from build123d import *

# Parameters (mm, degrees)
ESTRUSIONE_ESTRUSIONE1_DEPTH           = 20
SCHIZZO2_R                             = 3.15
TAGLIO_ESTRUSIONE1_DEPTH               = 0.5
FORO_SVASATO_PER_VITE_M3_1_D           = 3.4
FORO_SVASATO_PER_VITE_M3_1_CSINK_D     = 6.3
FORO_SVASATO_PER_VITE_M3_1_CSINK_ANGLE = 90


with BuildPart() as part:
    # Schizzo1 → Estrusione-Estrusione1 (new body)
    with BuildSketch(Plane.XY):
        with BuildLine():
            Line((7.2, -12.4), (-7.2, -12.4))
            Line((-7.2, -12.4), (-7.2, -15.4))
            ThreePointArc((-7.2, -15.4), (0, -16.607910427), (7.2, -15.4))
            Line((7.2, -15.4), (7.2, -12.4))
        make_face()
    extrude(amount=-ESTRUSIONE_ESTRUSIONE1_DEPTH)

    # Schizzo2 → Taglio-Estrusione1 (cut)
    with BuildSketch(Plane(origin=(0, -16.607910427, 0), x_dir=(-1, 0, 0), z_dir=(0, -1, 0))):
        with Locations((0, 13.333333333)):
            Circle(SCHIZZO2_R)
        with Locations((0, 6.666666667)):
            Circle(SCHIZZO2_R)
    extrude(amount=-TAGLIO_ESTRUSIONE1_DEPTH, mode=Mode.SUBTRACT)

    # Foro svasato per Vite M3-1 (through all)
    with Locations(Plane(origin=(0, -16.107910427, -6.666666667), x_dir=(-1, 0, 0), z_dir=(0, -1, 0))):
        with Locations((0, 0), (0, 6.666666666)):
            CounterSinkHole(FORO_SVASATO_PER_VITE_M3_1_D / 2, FORO_SVASATO_PER_VITE_M3_1_CSINK_D / 2, counter_sink_angle=FORO_SVASATO_PER_VITE_M3_1_CSINK_ANGLE)


solid = part.part
Part model, mm, in its own coordinate system. A direction names the side the tool comes from. Coordinates: 2 decimals unless noted, no trailing zeros. Loops run counter-clockwise (first coordinate to the right, second up) from the corner with the lowest first, then second, coordinate; pieces in that order, holes last. Notation, with made-up numbers: (-18, 86) - (22, 86) arc R11 ccw to (22, 100) - close; hole circle Ø2 at (-8.5, 37.25). An arc over 180 degrees is marked (long way). Write each question's results on one line, items separated by ' | '. Start each with the question number.
Q1. Slice it at B-B on y = -12.8. Give the cut face in (x, z), and give its area (3 significant figures).
Q2. Two-plate mould, pull along X, no slides. Class faces 1 (the cylindrical face through (-1.73, -16.54, -9.86)), 2 (the cylindrical face through (-0.369, -13.513, -11.674)), 3 (the flat face through (0, -12.4, -10)): +X half, -X half, draft (parallel to the pull), parting line (faces both ways), or undercut.
Q3. Slice it at A-A on x = 0. Give the cut face in (y, z), and give its area (3 significant figures).
Q4. Slice it at C-C on x = 4. Give the cut face in (y, z), and give its area (3 significant figures).
Q5. Drop flat-ended pins along their axis: pin 1 Ø4 at (x, z) = (0, -6.67) entering from -Y; pin 2 Ø1.5 at (x, z) = (-3, -13) entering from -Y; pin 3 Ø5.5 at (x, z) = (0, -13.33) entering from -Y. Give the stop position or say it passes through.
Q6. Slice it at D-D on x = -4.75. Give the cut face in (y, z), and give its area (3 significant figures).
Q7. Probe line 1 along Z through (x, y) = (0, -16.2); line 2 along Z through (x, y) = (0, -13.2); line 3 along X through (y, z) = (-12.8, -13). List the from-to ranges inside material, lowest first.
Q8. Which spindle directions (+Z, -Z, +X, -X, +Y, -Y) get a long thin tool onto all of the face, cutting with end or side? Do faces 4 (the flat face through (0, -14, -20)), 5 (the cylindrical face through (2.32, -16.31, -8.8)). Say none if no direction does.
Answer:
1) outline: (-7.2, -20) - (7.2, -20) - (7.2, 0) - (-7.2, 0) - close; hole circle Ø3.4 at (0, -13.33); hole circle Ø3.4 at (0, -6.67) | area: 270 mm2
2) face 1: parting line | face 2: undercut | face 3: draft
3) outline: (-16.61, -20) - (-12.4, -20) - (-12.4, -15.03) - (-14.66, -15.03) - (-16.11, -16.48) - (-16.61, -16.48) - close; (-16.61, -10.18) - (-16.11, -10.18) - (-14.66, -11.63) - (-12.4, -11.63) - (-12.4, -8.37) - (-14.66, -8.37) - (-16.11, -9.82) - (-16.61, -9.82) - close; (-16.61, -3.52) - (-16.11, -3.52) - (-14.66, -4.97) - (-12.4, -4.97) - (-12.4, 0) - (-16.61, 0) - close | area: 48.4 mm2
4) outline: (-16.24, -20) - (-12.4, -20) - (-12.4, 0) - (-16.24, 0) - close | area: 76.8 mm2
5) pin 1: stops at y = -14.96 | pin 2: stops at y = -16.41 | pin 3: stops at y = -15.71
6) outline: (-16.09, -20) - (-12.4, -20) - (-12.4, 0) - (-16.09, 0) - close | area: 73.8 mm2
7) line 1: z = -20 to -16.48, -10.18 to -9.82, -3.52 to 0 | line 2: z = -20 to -15.03, -11.63 to -8.37, -4.97 to 0 | line 3: x = -7.2 to -1.67, 1.67 to 7.2
8) face 4: -Z, +X, -X, +Y, -Y | face 5: -Y
